from build123d import *

# Parameters (mm, degrees)
F0_R     = 40
F0_R_2   = 30
F1_DEPTH = 20
F2_R     = 40
F2_R_2   = 30
F3_DEPTH = 10
F4_R     = 20
F5_DEPTH = 10
F6_R     = 5
F7_DEPTH = 25
F8_R     = 4.99999
F9_R     = 5


# Not quite as in the source:
# - a fillet or chamfer is up to 0.001 mm smaller than in the source, because OpenCascade refuses the exact size


with BuildPart() as f1:
    # F0 (on Front) → F1 (new body)
    with BuildSketch(Plane.XZ):
        Circle(F0_R)
        Circle(F0_R_2, mode=Mode.SUBTRACT)
    extrude(amount=F1_DEPTH)

    # F2 (on face) → F3 (join)
    with BuildSketch(Plane.XZ.offset(20)):
        Circle(F2_R)
        Circle(F2_R_2, mode=Mode.SUBTRACT)
        Circle(F2_R_2)
    extrude(amount=F3_DEPTH)

    # F4 (on face) → F5 (join)
    with BuildSketch(Plane.XZ.offset(30)):
        Circle(F4_R)
    extrude(amount=F5_DEPTH)

    # F6 (on face) → F7 (join)
    with BuildSketch(Plane.XZ.offset(40)):
        Circle(F6_R)
    extrude(amount=F7_DEPTH)

    # F8 (radius 5 in the source; OpenCascade refuses exactly that, so slightly less here)
    f8_edges = [f1.edges().sort_by_distance(p)[0] for p in [
        (-20, -30, 0),
        (-20, -40, 0),
    ]]
    fillet(f8_edges, radius=F8_R)

    # F9
    f9_edges = [f1.edges().sort_by_distance(p)[0] for p in [
        (-40, -30, 0),
    ]]
    fillet(f9_edges, radius=F9_R)


solid = f1.part
CAD build for the part. Positions are in the model's coordinates, mm. A direction names the side the tool comes from. Coordinates: 2 decimals unless noted, no trailing zeros. Order: outer loops, then holes, each group sorted by start corner. A loop starts at its lowest first (then second) coordinate and runs counter-clockwise, first axis right, second up.
Item 1: Pin check, flat tips, straight feed: pin 1 Ø8 at (x, z) = (-17, 10.5) entering from -Y; pin 2 Ø9 at (x, z) = (-7, 6.5) entering from -Y; pin 3 Ø8 at (x, z) = (30.5, 30.5) entering from +Y; pin 4 Ø1 at (x, z) = (11, 14) entering from +Y. Stop position of each tip, or through.
Check sheet entries:
pin 1: stops at y = -39.9
pin 2: stops at y = -40
pin 3: stops at y = 0
pin 4: stops at y = -20
Item 2: 3-axis set-ups, long thin cutter, end or side, ignore diameter. For faces 1 (the face through (-29.97, -9.86, 1.32)), 2 (the face through (-24, -30, 8)), 3 (the face through (6, 0, 30)): which of +Z, -Z, +X, -X, +Y, -Y reach the whole face in a straight line?
Check sheet entries:
face 1: +Y
face 2: -Y
face 3: +Z, -Z, +X, -X, +Y
Item 3: Two-plate mould, pull along X, no slides. Class faces 4 (the face through (-8.67, -12.32, -39.05)), 5 (the face through (-4, -40, 4)), 6 (the face through (0, -20, 0)): +X half, -X half, draft (parallel to the pull), parting line (faces both ways), or undercut.
Check sheet entries:
face 4: parting line
face 5: draft
face 6: undercut
Item 4: Band-saw the part on D-D on y = -23.5. List the corners of the cut face in (x, z), plus the area to 3 significant figures.
Check sheet entries:
outline: circle Ø80 at (0, 0)
area: 5,030 mm2
Item 5: Drill centre lines: L1, parallel to Z at x = 0, y = -12.5; L2, parallel to Y at x = 8, z = 28; L3, parallel to Y at x = -9, z = -1.5. Where is each one in solid material? Low to high.
Check sheet entries:
L1: z = -40 to -30, 30 to 40
L2: y = -30 to -20
L3: y = -40 to -20
Item 6: Band-saw the part on B-B on y = -4.5. List the corners of the cut face in (x, z), plus the area to 3 significant figures.
Check sheet entries:
outline: circle Ø80 at (0, 0); hole circle Ø60 at (0, 0)
area: 2,200 mm2
